Answer from the drawing. Dimensions are ordinates in mm from the lowest x, y and z of the part. Coordinates: 2 decimals unless noted, no trailing zeros. Loops run counter-clockwise (first coordinate to the right, second up) from the corner with the lowest first, then second, coordinate; pieces in that order, holes last.
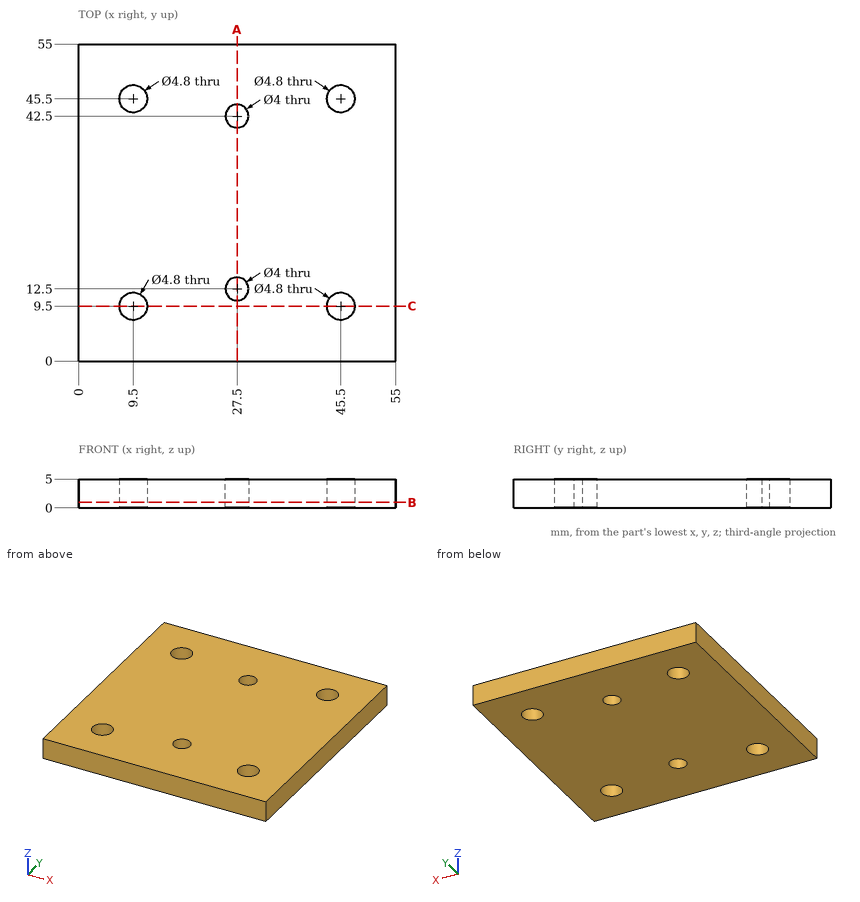
Item 1: A cutting plane is placed at A-A on x = 27.5. Determine the outline of the cut face in (y, z).
Numbers:
outline: (0, 0) - (10.5, 0) - (10.5, 5) - (0, 5) - close; (14.5, 0) - (40.5, 0) - (40.5, 5) - (14.5, 5) - close; (44.5, 0) - (55, 0) - (55, 5) - (44.5, 5) - close
Item 2: Find the intervals of material crossed by line 1 along Y through (x, z) = (27.5, 2.5); line 2 along Y through (x, z) = (45.5, 2.5), in increasing order.
Numbers:
line 1: y = 0 to 10.5, 14.5 to 40.5, 44.5 to 55
line 2: y = 0 to 7.1, 11.9 to 43.1, 47.9 to 55
Item 3: A cutting plane is placed at C-C on y = 9.5. Determine the outline of the cut face in (x, z), then the cut area to 3 significant figures.
Numbers:
outline: (0, 0) - (7.1, 0) - (7.1, 5) - (0, 5) - close; (11.9, 0) - (43.1, 0) - (43.1, 5) - (11.9, 5) - close; (47.9, 0) - (55, 0) - (55, 5) - (47.9, 5) - close
area: 227 mm2
Item 4: A cutting plane is placed at B-B on z = 0.95. Determine the outline of the cut face in (x, y).
Numbers:
outline: (0, 0) - (55, 0) - (55, 55) - (0, 55) - close; hole circle Ø4.8 at (9.5, 9.5); hole circle Ø4.8 at (9.5, 45.5); hole circle Ø4 at (27.5, 12.5); hole circle Ø4 at (27.5, 42.5); hole circle Ø4.8 at (45.5, 9.5); hole circle Ø4.8 at (45.5, 45.5)
